```python
from build123d import *

# Parameters (mm, degrees)
SKETCH2_R               = 1.3375
BOSS_EXTRUDE2_DEPTH     = 25.4
SKETCH4_W               = 12.7
SKETCH4_H               = 12.7
CUT_EXTRUDE2_DEPTH      = 12.7
CUT_EXTRUDE3_DEPTH      = 110.534359325
CUT_EXTRUDE3_DEPTH_BACK = 110.534359325
SKETCH5_W               = 5.08
SKETCH5_H               = 6.35
CUT_EXTRUDE7_DEPTH      = 110.233274388


with BuildPart() as part:
    # Sketch2 → Boss-Extrude2 (new body)
    with BuildSketch(Plane.XY):
        with BuildLine():
            Line((-10.776857143, 6.112115909), (100.983142857, 6.112115909))
            ThreePointArc((100.983142857, 6.112115909), (106.063142857, 1.032115909), (100.983142857, -4.047884091))
            Line((100.983142857, -4.047884091), (-10.776857143, -4.047884091))
            ThreePointArc((-10.776857143, -4.047884091), (-15.856857143, 1.032115909), (-10.776857143, 6.112115909))
        make_face()
        with Locations((-10.776857143, 1.032115909)):
            Circle(SKETCH2_R, mode=Mode.SUBTRACT)
        with Locations((100.983142857, 1.032115909)):
            Circle(SKETCH2_R, mode=Mode.SUBTRACT)
    extrude(amount=BOSS_EXTRUDE2_DEPTH)

    # Sketch4 → Cut-Extrude2 (cut)
    with BuildSketch(Plane(origin=(0, 6.112115909, 0), x_dir=(1, 0, 0), z_dir=(0, 1, 0))):
        with Locations((-9.506857143, -12.7)):
            Rectangle(SKETCH4_W, SKETCH4_H)
    extrude(amount=-CUT_EXTRUDE2_DEPTH, mode=Mode.SUBTRACT)

    # Sketch5 → Cut-Extrude3 (cut, two sides: drawn at the far end of the back side and taken through both)
    with BuildSketch(Plane(origin=(0, 6.112115909, 0), x_dir=(1, 0, 0), z_dir=(0, 1, 0)).offset(-CUT_EXTRUDE3_DEPTH_BACK)):
        Polygon((87.013142857, 0), (3.193142857, 0), (14.191665485, -6.35), (100.983142857, -6.35), (100.983142857, 0), align=None)
        Polygon((100.983142857, -25.4), (100.983142857, -19.05), (14.191665485, -19.05), (3.193142857, -25.4), (87.013142857, -25.4), align=None)
        with Locations((103.523142857, -22.225)):
            Rectangle(SKETCH5_W, SKETCH5_H)
        with Locations((103.523142857, -3.175)):
            Rectangle(SKETCH5_W, SKETCH5_H)
    extrude(amount=CUT_EXTRUDE3_DEPTH + CUT_EXTRUDE3_DEPTH_BACK, mode=Mode.SUBTRACT)

    # Sketch13 → Cut-Extrude7 (cut, through all)
    with BuildSketch(Plane.XY.offset(25.4)):
        Polygon((87.013142857, 6.112115909), (76.014620229, 3.572115909), (14.191665485, 3.572115909), (3.193142857, 6.112115909), align=None)
        Polygon((87.013142857, -4.047884091), (3.193142857, -4.047884091), (14.191665485, -1.507884091), (76.014620229, -1.507884091), align=None)
    extrude(amount=-CUT_EXTRUDE7_DEPTH, mode=Mode.SUBTRACT)


solid = part.part
```
Build history of the part. All positions in model axes, mm. A direction names the side the tool comes from. Give positions to 0.01 mm unless a question says otherwise; leave off trailing zeros. Loops run counter-clockwise (first coordinate to the right, second up) from the corner with the lowest first, then second, coordinate; pieces in that order, holes last.
1) Band-saw the part on B-B on x = 49.5. List the corners of the cut face in (y, z).
Values follow:
outline: (-1.51, 6.35) - (3.57, 6.35) - (3.57, 19.05) - (-1.51, 19.05) - close
2) Band-saw the part on D-D on x = 93. List the corners of the cut face in (y, z), then the cut area to 3 significant figures.
Values follow:
outline: (-4.05, 6.35) - (6.11, 6.35) - (6.11, 19.05) - (-4.05, 19.05) - close
area: 129 mm2
3) Drop flat-ended pins along their axis: P1, Ø4, axis at y = -1.5, z = 6, coming from the -X side; P2, Ø6, axis at x = 63.5, y = -2.5, coming from the +Z side; P3, Ø3.5, axis at x = -10.78, y = 1.03, coming from the +Z side; P4, Ø1.6, axis at x = -10.78, y = 1.03, coming from the -Z side. Give the stop position or say it passes through.
Values follow:
P1: stops at x = -15.83
P2: stops at z = 19.05
P3: stops at z = 25.4
P4: passes through
4) Probe line 1 along Z through (x, y) = (-10, -2.25); line 2 along Y through (x, z) = (36, 15.75); line 3 along Z through (x, y) = (51, 2). List the from-to ranges inside material, lowest first.
Values follow:
line 1: z = 0 to 6.35, 19.05 to 25.4
line 2: y = -1.51 to 3.57
line 3: z = 6.35 to 19.05
5) Band-saw the part on A-A on z = 5.25. List the corners of the cut face in (x, y) (1 decimal).
Values follow:
outline: (-10.8, -4) - (3.2, -4) - (12.3, -1.9) - (12.3, 4) - (3.2, 6.1) - (-10.8, 6.1) arc R5.1 ccw to start; hole circle Ø2.7 at (-10.8, 1)
6) Band-saw the part on C-C on z = 12.25. List the corners of the cut face in (x, y) (1 decimal).
Values follow:
outline: (-3.2, -4) - (3.2, -4) - (14.2, -1.5) - (76, -1.5) - (87, -4) - (101, -4) arc R5.1 ccw to (101, 6.1) - (87, 6.1) - (76, 3.6) - (14.2, 3.6) - (3.2, 6.1) - (-3.2, 6.1) - close; hole circle Ø2.7 at (101, 1)
7) Two-plate mould, pull along X, no slides. Class faces 1 (the face through (-12.113, 1.091, 22.181)), 2 (the face through (-15.856, 0.92, 22.181)), 3 (the face through (-2, 6.112, 13)): released by +X, released by -X, zero draft, split by the parting line, or undercut.
Values follow:
face 1: undercut
face 2: released by -X
face 3: zero draft
8) 3-axis set-ups, long thin cutter, end or side, ignore diameter. For faces 4 (the face through (8, 5, 13)), 5 (the face through (61, 1, 19.05)), 6 (the face through (7.39, -3.08, 12.88)), 7 (the face through (59, 1, 6.35)): which of +Z, -Z, +X, -X, +Y, -Y reach the whole face in a straight line?
Values follow:
face 4: +Z, -Z, +Y
face 5: +Z, +X, +Y, -Y
face 6: +Z, -Z, -Y
face 7: -Z, +X, +Y, -Y
